```python
from build123d import *

# Parameters (mm, degrees)
PAD_DEPTH    = 18
SKETCH001_W  = 18
SKETCH001_H  = 60
POCKET_DEPTH = 12
CHAMFER_SIZE = 15
FILLET_R     = 5
FILLET001_R  = 15
FILLET002_R  = 50


with BuildPart() as part:
    # Sketch → Pad (new body)
    with BuildSketch(Plane.XY):
        Polygon((0, 185), (0, -185), (78.33092, -173.991307), (110, -25), (110, 25), (78.33092, 173.991307), align=None)
    extrude(amount=PAD_DEPTH)

    # Sketch001 → Pocket (cut)
    with BuildSketch(Plane.XY.offset(18)):
        with Locations((55, 0)):
            Rectangle(SKETCH001_W, SKETCH001_H)
    extrude(amount=-POCKET_DEPTH, mode=Mode.SUBTRACT)

    # Chamfer
    chamfer_edges = [part.edges().sort_by_distance(p)[0] for p in [
        (0, -185, 9),
        (0, 185, 9),
    ]]
    chamfer(chamfer_edges, length=CHAMFER_SIZE)

    # Fillet
    fillet_edges = [part.edges().sort_by_distance(p)[0] for p in [
        (14.854021, 182.912403, 9),
        (0, 170, 9),
        (0, -170, 9),
        (14.854021, -182.912403, 9),
    ]]
    fillet(fillet_edges, radius=FILLET_R)

    # Fillet001
    fillet001_edges = [part.edges().sort_by_distance(p)[0] for p in [
        (78.33092, -173.991307, 9),
        (78.33092, 173.991307, 9),
    ]]
    fillet(fillet001_edges, radius=FILLET001_R)

    # Fillet002
    fillet002_edges = [part.edges().sort_by_distance(p)[0] for p in [
        (110, -25, 9),
        (110, 25, 9),
    ]]
    fillet(fillet002_edges, radius=FILLET002_R)


solid = part.part
```
Model file for the job. Use its own axes, mm. A direction names the side the tool comes from. Coordinates: 2 decimals unless noted, no trailing zeros. Write each loop counter-clockwise with the first axis right and the second up, starting at its lowest first coordinate (ties: lowest second). Pieces come first, ordered by that corner, then holes. Notation, with made-up numbers: (89.5, 68.5) - (108.5, 68.5) arc R18 cw to (108.5, 101.5) - close; hole circle Ø7 at (45.25, 80). An arc over 180 degrees is marked (long way). One line per item, written item: value. Start each with the question number.
1. Probe line 1 (Y direction, x = 60, z = 13.5); line 2 (X direction, y = -28.5, z = 6.75); line 3 (X direction, y = -26, z = 16.75). List the from-to ranges inside material, lowest first. Write a range as from..to.
2. Slice it at B-B (y = 3). Write the cut outline in (x, z).
3. Slice it at D-D (y = -127.5). Write the cut outline in (x, z), plus the area to 3 significant figures.
4. Slice it at A-A (z = 15). Write the cut outline in (x, y), plus the area to 3 significant figures.
5. Flat gauge pins, fed straight in: pin 1 (9 mm diameter, centred on x = 59, y = 8.5, fed in from +Z); pin 2 (4 mm diameter, centred on x = 94.5, y = 69.5, fed in from -Z); pin 3 (4 mm diameter, centred on x = 23.5, z = 5, fed in from -Y); pin 4 (6 mm diameter, centred on x = 52.5, z = 11, fed in from +Y). Where does each tip first touch, or does it go through?
6. Slice it at C-C (x = 40.5). Write the cut outline in (y, z).
7. Tool access for faces 1 (the flat face through (46, 0, 12)), 2 (the cylindrical face through (109.734, -24.898, 9.126)): list every direction of +Z, -Z, +X, -X, +Y, -Y with a clear straight run to the whole face (end or side of a thin tool).
Answers below:
1. line 1: y = -176.57..-30, 30..176.57
1. line 2: x = 0..46, 64..109.23
1. line 3: x = 0..46, 64..109.61
2. outline: (0, 0) - (110, 0) - (110, 18) - (64, 18) - (64, 6) - (46, 6) - (46, 18) - (0, 18) - close
3. outline: (0, 0) - (88.21, 0) - (88.21, 18) - (0, 18) - close
3. area: 1,590 mm^2
4. outline: (0, -167.72) arc R5 ccw to (1.72, -171.49) - (13.13, -181.42) arc R5 ccw to (17.11, -182.6) - (67.93, -175.45) arc R15 ccw to (80.51, -163.72) - (108.91, -30.14) arc R50 ccw to (110, -19.74) - (110, 19.74) arc R50 ccw to (108.91, 30.14) - (80.51, 163.72) arc R15 ccw to (67.93, 175.45) - (17.11, 182.6) arc R5 ccw to (13.13, 181.42) - (1.72, 171.49) arc R5 ccw to (0, 167.72) - close; hole (46, -30) - (64, -30) - (64, 30) - (46, 30) - close
4. area: 33,100 mm^2
5. pin 1: stops at z = 6
5. pin 2: stops at z = 0
5. pin 3: stops at y = -181.98
5. pin 4: stops at y = 178.04
6. outline: (-179.31, 0) - (179.31, 0) - (179.31, 18) - (-179.31, 18) - close
7. face 1: +Z
7. face 2: +Z, -Z, +X, -Y
